Autodesk Inventor part; units mm, degrees
ref_plane "YZ Plane" through (0, 0, 0) normal (1, 0, 0) x (0, 1, 0)
ref_plane "XZ Plane" through (0, 0, 0) normal (0, 1, 0) x (-1, 0, 0)
ref_plane "XY Plane" through (0, 0, 0) normal (0, 0, 1) x (1, 0, 0)
sketch "Sketch1" plane through (0, 0, 0) normal (0, 0, 1) x (1, 0, 0)
  circle A0 centre (9.0035, 0) radius 6
  circle A1 centre (-10.4965, 0) radius 6
  line L0 (-16.4965, 0) -> (-25.4965, 0)
  line L1 (-25.4965, 0) -> (-25.4965, 10)
  line L2 (-25.4965, 10) -> (24.0035, 10)
  line L3 (24.0035, 10) -> (24.0035, 0)
  line L4 (24.0035, 0) -> (15.0035, 0)
  line L5 (-4.4965, 0) -> (3.0035, 0)
  point P0 (0, 0)
  dimension "d4" = 12
  dimension "d5" = 12
  dimension "d6" = 19.5
  dimension "d7" = 0
  dimension "d8" = 0
  dimension "d9" = 9
  dimension "d10" = 9
  dimension "d11" = 10
  dimension "d12" = 0
extrude "Extrusion1" add sketch "Sketch1" along normal blind 38 contours A0 L5 A1 L0 L1 L2 L3 L4
sketch "Sketch2" plane through (-4.4965, 0, 0) normal (0, -1, 0) x (1, 0, 0)
  line L0 (-21, 0) -> (-12, 0)
  line L1 (-12, 0) -> (-12, 38)
  line L2 (-21, 38) -> (-12, 38)
  line L3 (-21, 0) -> (-21, 38)
  line L4 (0, 0) -> (7.5, 0)
  line L5 (7.5, 0) -> (7.5, 38)
  line L6 (0, 38) -> (7.5, 38)
  line L7 (0, 0) -> (0, 38)
  line L8 (19.5, 0) -> (28.5, 0)
  line L9 (28.5, 0) -> (28.5, 38)
  line L10 (19.5, 38) -> (28.5, 38)
  line L11 (19.5, 0) -> (19.5, 38)
  line L12 (-21, 0) -> (-12, 0)
  line L13 (-21, 0) -> (0, 0)
  line L14 (-21, 9.5) -> (0, 9.5)
  line L15 (-21, 28.5) -> (0, 28.5)
  line L16 (0, 0) -> (0, 38)
  line L17 (-12, 38) -> (0, 38)
  line L18 (-21, 38) -> (0, 38)
  point P0 (4.4965, 0)
  dimension "d17" = 19
  dimension "d18" = 9.5
extrude "Extrusion2" cut sketch "Sketch2" against normal through all contours L3 L14 L1 L0 | L1 L14 L7 L13 | L3 L2 L1 L15 | L1 L17 L7 L15
fillet "Fillet1" radius 5 2 edges at (-4.4965, 5, 28.5) (-4.4965, 5, 9.5)
fillet "Fillet2" radius 3 2 edges at (-4.4965, 5, 0) (-4.4965, 5, 38)
fillet "Fillet2" radius 1 2 edges at (24.0035, 5, 38) (24.0035, 5, 0)
fillet "Fillet2" radius 2 2 edges at (-25.4965, 5, 9.5) (-25.4965, 5, 28.5)
sketch "Sketch3" plane through (3.0035, 0, 0) normal (0, -1, 0) x (1, 0, 0)
  arc A0 (-28.5, 11.5) -> (-26.5, 9.5) centre (-26.5, 11.5) ccw
  line L0 (-26.5, 9.5) -> (-19.5, 9.5)
  line L1 (-19.5, 9.5) -> (-19.5, 28.5)
  line L2 (-19.5, 28.5) -> (-26.5, 28.5)
  arc A1 (-26.5, 28.5) -> (-28.5, 26.5) centre (-26.5, 26.5) ccw
  line L3 (-28.5, 11.5) -> (-28.5, 26.5)
  arc A2 (-4.5, 38) -> (-7.5, 35) centre (-4.5, 35) ccw
  line L4 (-7.5, 33.5) -> (-7.5, 35)
  line L5 (-7.5, 4.5) -> (-7.5, 33.5)
  line L6 (-7.5, 3) -> (-7.5, 4.5)
  arc A3 (-7.5, 3) -> (-4.5, 0) centre (-4.5, 3) ccw
  line L7 (-4.5, 0) -> (0, 0)
  line L8 (0, 0) -> (0, 38)
  line L9 (-4.5, 38) -> (0, 38)
  arc A4 (21, 37) -> (20, 38) centre (20, 37) ccw
  line L10 (12, 38) -> (20, 38)
  line L11 (12, 0) -> (12, 38)
  line L12 (12, 0) -> (20, 0)
  arc A5 (20, 0) -> (21, 1) centre (20, 1) ccw
  line L13 (21, 1) -> (21, 37)
  point P0 (-3.0035, 0)
  point P1 (-3.75, 4.5)
  point P2 (-3.75, 19)
  point P3 (-3.75, 33.5)
  point P4 (16.5, 4.5)
  point P5 (16.5, 19)
  point P6 (16.5, 33.5)
  point P7 (-24, 19)
  dimension "d23" = 7.5
  dimension "d24" = 3.75
  dimension "d25" = 9
  dimension "d26" = 4.5
  dimension "d27" = 9
  dimension "d28" = 4.5
  dimension "d29" = 19
  dimension "d30" = 9.5
  dimension "d31" = 4.5
  dimension "d32" = 4.5
hole "Hole1" at (-0.7465, 0, 4.5) at (-0.7465, 0, 19) at (-0.7465, 0, 33.5) at (19.5035, 0, 4.5) at (19.5035, 0, 19) at (19.5035, 0, 33.5) at (-20.9965, 0, 19) direction (0, 1, 0) diameter 3 end through all
sketch "Sketch4" plane through (24.0035, 0, 1) normal (1, 0, 0) x (0, 0, -1)
  line L0 (-16.5, 10) -> (-16.5, 0)
  line L1 (-19.5, 10) -> (-19.5, 0)
  line L2 (-31, 10) -> (-31, 0)
  line L3 (-5, 10) -> (-5, 0)
  line L4 (0, 10) -> (0, 0)
  line L5 (0, 10) -> (-36, 10)
  line L6 (-36, 0) -> (-36, 10)
  line L7 (0, 0) -> (-36, 0)
  point P0 (1, 0)
  point P1 (-25.25, 5)
  point P2 (-10.75, 5)
  dimension "d41" = 11.5
  dimension "d42" = 11.5
  dimension "d43" = 5.75
  dimension "d44" = 5.75
  dimension "d45" = 10
  dimension "d46" = 5
hole "Hole2" at (24.0035, 5, 26.25) at (24.0035, 5, 11.75) direction (-1, 0, 0) diameter 2.5 depth 8 tip angle 118
properties part number "3DP_PLA_X_axis_carriage_half" material "ABS Plastic"
The listing builds one solid part. Answer for the finished solid, in the listing's coordinates (mm). A direction names the side the tool comes from. Coordinates: 2 decimals unless noted, no trailing zeros. Write each loop counter-clockwise with the first axis right and the second up, starting at its lowest first coordinate (ties: lowest second). Pieces come first, ordered by that corner, then holes.
Q1. Which of the six approach directions +Z, -Z, +X, -X, +Y, -Y give full straight-line access (tool end or side, diameter ignored) to faces 4 (the cylindrical face through (20, 5, 25)), 5 (the cylindrical face through (20.416, 5.07, 34.69))?
Returned:
face 4: +X
face 5: +Y, -Y
Q2. Section D-D, the plane y = 9 is taken. Write down the section's boundary in (x, z), then the cut area to 3 significant figures.
Returned:
outline: (-25.5, 11.5) arc R2 ccw to (-23.5, 9.5) - (-9.5, 9.5) arc R5 cw to (-4.5, 4.5) - (-4.5, 3) arc R3 ccw to (-1.5, 0) - (23, 0) arc R1 ccw to (24, 1) - (24, 37) arc R1 ccw to (23, 38) - (-1.5, 38) arc R3 ccw to (-4.5, 35) - (-4.5, 33.5) arc R5 cw to (-9.5, 28.5) - (-23.5, 28.5) arc R2 ccw to (-25.5, 26.5) - close; hole circle Ø3 at (-21, 19); hole circle Ø3 at (-0.75, 4.5); hole circle Ø3 at (-0.75, 19); hole circle Ø3 at (-0.75, 33.5); hole circle Ø3 at (19.5, 4.5); hole circle Ø3 at (19.5, 19); hole circle Ø3 at (19.5, 33.5)
area: 1,440 mm2
Q3. Given P1, Ø2.5, axis at x = 19.5, z = 4.5, coming from the +Y side; P2, Ø3, axis at x = -18.5, y = 4, coming from the -Z side; P3, Ø1.2, axis at y = 3.5, z = 34, coming from the -X side; P4, Ø3, axis at x = -19.5, y = 5, coming from the +Z side, each flat-ended and moving along its own axis, determine where each tip first touches the part or whether it passes through.
Returned:
P1: passes through
P2: stops at z = 9.5
P3: stops at x = -4.5
P4: stops at z = 28.5
Q4. Section A-A, the plane y = 2 is taken. Give the number of separate pieces and of enclosed holes in the cut face, then the cut area to 3 significant figures.
Returned:
separate pieces: 3
enclosed holes: 7
area: 784 mm2
Q5. The mould has two halves that part along X. Classify faces 1 (the cylindrical face through (-10.6, 6, 18.8)), 2 (the cylindrical face through (23.703, 4.93, 0.285)), 3 (the flat face through (11, 6, 38)): released by +X, released by -X, zero draft, split by the parting line, or undercut.
Returned:
face 1: undercut
face 2: released by +X
face 3: zero draft
Q6. Find the intervals of material crossed by line 1 along X through (y, z) = (9, 33.5); line 2 along X through (y, z) = (7.25, 19); line 3 along X through (y, z) = (1.5, 16.5), in increasing order.
Returned:
line 1: x = -4.5 to -2.25, 0.75 to 18, 21 to 24
line 2: x = -25.5 to -22.5, -19.5 to -2.25, 0.75 to 18, 21 to 24
line 3: x = -25.5 to -16.31, -4.69 to 3.19, 14.81 to 24
Q7. Section C-C, the plane z = 22.5 is taken. Write down the section's boundary in (x, y).
Returned:
outline: (-25.5, 0) - (-16.5, 0) arc R6 cw to (-4.5, 0) - (3, 0) arc R6 cw to (15, 0) - (24, 0) - (24, 10) - (-25.5, 10) - close
Q8. Section B-B, the plane x = 17 is taken. Write down the section's boundary in (y, z).
Returned:
outline: (0, 0) - (10, 0) - (10, 38) - (0, 38) - close; hole circle Ø2.5 at (5, 11.75); hole circle Ø2.5 at (5, 26.25)
